The listing builds one solid part. Answer for the finished solid, in the listing's coordinates (mm). Face numbers are marked on the shaded views. A direction names the side the tool comes from. Coordinates: 2 decimals unless noted, no trailing zeros. Order: outer loops, then holes, each group sorted by start corner. A loop starts at its lowest first (then second) coordinate and runs counter-clockwise, first axis right, second up. Notation, with made-up numbers: (-28, 15.5) -> (-17, 15.5) arc R28 ccw to (-17, 53.5) -> close; hole circle Ø11 at (86, -38). An arc over 180 degrees is marked (long way). Return JSON: item names as keys, results as strings.
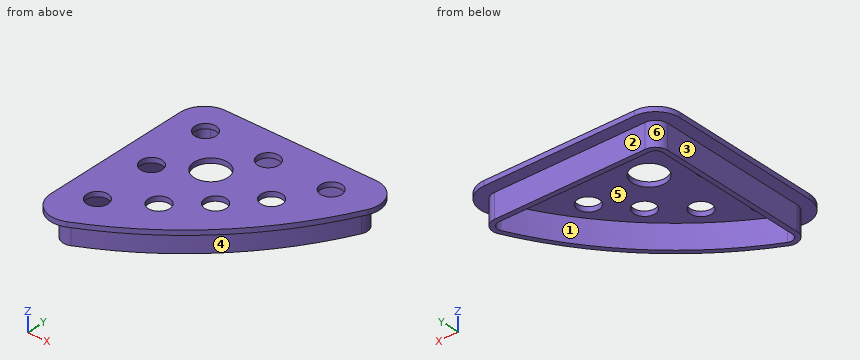
from build123d import *

# Parameters (mm, degrees)
F1_DEPTH = 12.7
F3_DEPTH = 2.54
F4_R     = 5.588
F4_R_2   = 8.763
F5_DEPTH = 25.4


with BuildPart() as f1:
    # F0 (on Top) → F1 (new body)
    with BuildSketch(Plane.XY):
        with BuildLine():
            ThreePointArc((0.508, -85.5526443698), (3.4826484531, -90.931259613), (9.6196541528, -91.2706655607))
            ThreePointArc((9.6196541528, -91.2706655607), (57.3578547677, -57.3578547677), (91.2706655607, -9.6196541528))
            ThreePointArc((91.2706655607, -9.6196541528), (90.931259613, -3.4826484531), (85.5526443698, -0.508))
            Line((85.5526443698, -0.508), (6.858, -0.508))
            ThreePointArc((6.858, -0.508), (2.3678719395, -2.3678719395), (0.508, -6.858))
            Line((0.508, -6.858), (0.508, -85.5526443698))
        make_face()
        with BuildLine():
            ThreePointArc((88.9834570843, -8.5149924917), (55.5618035435, -55.5618035435), (8.5149924917, -88.9834570843))
            ThreePointArc((8.5149924917, -88.9834570843), (4.8327890719, -88.7798135157), (3.048, -85.5526443698))
            Line((3.048, -85.5526443698), (3.048, -6.858))
            ThreePointArc((3.048, -6.858), (4.1639231637, -4.1639231637), (6.858, -3.048))
            Line((6.858, -3.048), (85.5526443698, -3.048))
            ThreePointArc((85.5526443698, -3.048), (88.7798135157, -4.8327890719), (88.9834570843, -8.5149924917))
        make_face(mode=Mode.SUBTRACT)
    extrude(amount=F1_DEPTH)

    # F2 (on face) → F3 (join)
    with BuildSketch(Plane.XY.offset(12.7)):
        with BuildLine():
            Line((85.5526443698, 5.842), (6.858, 5.842))
            ThreePointArc((6.858, 5.842), (-2.1222561211, 2.1222561211), (-5.842, -6.858))
            Line((-5.842, -6.858), (-5.842, -85.5526443698))
            ThreePointArc((-5.842, -85.5526443698), (0.1072969063, -96.3098748563), (12.3813083055, -96.9886867517))
            ThreePointArc((12.3813083055, -96.9886867517), (61.8479828282, -61.8479828282), (96.9886867517, -12.3813083055))
            ThreePointArc((96.9886867517, -12.3813083055), (96.3098748563, -0.1072969063), (85.5526443698, 5.842))
        make_face()
        with BuildLine():
            ThreePointArc((9.6196541528, -91.2706655607), (3.4826484531, -90.931259613), (0.508, -85.5526443698))
            Line((0.508, -85.5526443698), (0.508, -6.858))
            ThreePointArc((0.508, -6.858), (2.3678719395, -2.3678719395), (6.858, -0.508))
            Line((6.858, -0.508), (85.5526443698, -0.508))
            ThreePointArc((85.5526443698, -0.508), (90.931259613, -3.4826484531), (91.2706655607, -9.6196541528))
            ThreePointArc((91.2706655607, -9.6196541528), (57.3578547677, -57.3578547677), (9.6196541528, -91.2706655607))
        make_face(mode=Mode.SUBTRACT)
        with BuildLine():
            Line((0.508, -6.858), (0.508, -85.5526443698))
            ThreePointArc((0.508, -85.5526443698), (3.4826484531, -90.931259613), (9.6196541528, -91.2706655607))
            ThreePointArc((9.6196541528, -91.2706655607), (57.3578547677, -57.3578547677), (91.2706655607, -9.6196541528))
            ThreePointArc((91.2706655607, -9.6196541528), (90.931259613, -3.4826484531), (85.5526443698, -0.508))
            Line((85.5526443698, -0.508), (6.858, -0.508))
            ThreePointArc((6.858, -0.508), (2.3678719395, -2.3678719395), (0.508, -6.858))
        make_face()
        with BuildLine():
            ThreePointArc((85.5526443698, -3.048), (88.7798135157, -4.8327890719), (88.9834570843, -8.5149924917))
            ThreePointArc((88.9834570843, -8.5149924917), (55.5618035435, -55.5618035435), (8.5149924917, -88.9834570843))
            ThreePointArc((8.5149924917, -88.9834570843), (4.8327890719, -88.7798135157), (3.048, -85.5526443698))
            Line((3.048, -85.5526443698), (3.048, -6.858))
            ThreePointArc((3.048, -6.858), (4.1639231637, -4.1639231637), (6.858, -3.048))
            Line((6.858, -3.048), (85.5526443698, -3.048))
        make_face(mode=Mode.SUBTRACT)
        with BuildLine():
            ThreePointArc((8.5149924917, -88.9834570843), (55.5618035435, -55.5618035435), (88.9834570843, -8.5149924917))
            ThreePointArc((88.9834570843, -8.5149924917), (88.7798135157, -4.8327890719), (85.5526443698, -3.048))
            Line((85.5526443698, -3.048), (6.858, -3.048))
            ThreePointArc((6.858, -3.048), (4.1639231637, -4.1639231637), (3.048, -6.858))
            Line((3.048, -6.858), (3.048, -85.5526443698))
            ThreePointArc((3.048, -85.5526443698), (4.8327890719, -88.7798135157), (8.5149924917, -88.9834570843))
        make_face()
    extrude(amount=F3_DEPTH)

    # F4 (on face) → F5 (cut)
    with BuildSketch(Plane.XY.offset(15.24)):
        with Locations((10.7421888637, -10.7421888637)):
            Circle(F4_R)
        with Locations((30.9239914141, -30.9239914141)):
            Circle(F4_R_2)
        with Locations((43.5884171282, -10.7421888637)):
            Circle(F4_R)
        with Locations((10.7421888637, -43.5884171282)):
            Circle(F4_R)
        with Locations((10.7421888637, -76.4346453927)):
            Circle(F4_R)
        with Locations((31.4632623863, -63.1055415565)):
            Circle(F4_R)
        with Locations((48.3775986466, -48.3775986466)):
            Circle(F4_R)
        with Locations((63.1055415565, -31.4632623863)):
            Circle(F4_R)
        with Locations((76.4346453927, -10.7421888637)):
            Circle(F4_R)
    extrude(amount=-F5_DEPTH, mode=Mode.SUBTRACT)


solid = f1.part
1. The part is cut by section C-C on y = -45.5. Give the vertices of the cut face in (x, z).
Answer block:
{"outline": "(-5.84, 12.7) -> (0.51, 12.7) -> (0.51, 0) -> (3.05, 0) -> (3.05, 12.7) -> (5.49, 12.7) -> (5.49, 15.24) -> (-5.84, 15.24) -> close; (15.99, 12.7) -> (43.59, 12.7) -> (43.59, 15.24) -> (15.99, 15.24) -> close; (53.17, 12.7) -> (64.86, 12.7) -> (64.86, 0) -> (68.18, 0) -> (68.18, 12.7) -> (76.34, 12.7) -> (76.34, 15.24) -> (53.17, 15.24) -> close"}
2. Each of these flat-tipped pins is pushed along its axis until it touches: pin 1 Ø2 at (x, z) = (45, 8) entering from -Y; pin 2 Ø6.5 at (y, z) = (-29.5, 7) entering from -X; pin 3 Ø14.5 at (x, y) = (48.38, -48.38) entering from -Z. Where does it stop, or does it pass through?
Answer block:
{"pin 1": "stops at y = -69.41", "pin 2": "stops at x = 0.51", "pin 3": "stops at z = 12.7"}
3. The part is cut by section A-A on z = 5.5. Give the vertices of the cut face in (x, y) (3 decimals).
Answer block:
{"outline": "(0.508, -85.553) arc R6.35 ccw to (9.62, -91.271) arc R175.379 ccw to (91.271, -9.62) arc R6.35 ccw to (85.553, -0.508) -> (6.858, -0.508) arc R6.35 ccw to (0.508, -6.858) -> close; hole (3.048, -85.553) arc R3.81 ccw to (8.515, -88.983) arc R172.839 ccw to (88.983, -8.515) arc R3.81 ccw to (85.553, -3.048) -> (6.858, -3.048) arc R3.81 ccw to (3.048, -6.858) -> close"}
4. For the marked faces 1, 2 and 3, determine the directions among +Z, -Z, +X, -X, +Y, -Y from which every point of the face is accessible in a straight line to the end or side of a thin tool.
Answer block:
{"face 1": "-Z", "face 2": "-Z, +X, -X, +Y", "face 3": "-Z, -X, +Y, -Y"}
5. Consider line 1 (Z direction, x = 18, y = -38.5); line 2 (X direction, y = -42.5, z = 12.75); line 3 (X direction, y = -14, z = 1.5). Determine where each line is inside the solid, lowest interval first. Write a range as from..to.
Answer block:
{"line 1": "z = 12.7..15.24", "line 2": "x = -5.84..5.26, 16.22..78.64", "line 3": "x = 0.51..3.05, 86.21..89.08"}
6. The part is cut by section B-B on x = 50.5. Give the vertices of the cut face in (y, z).
Answer block:
{"outline": "(-72.27, 12.7) -> (-63.86, 12.7) -> (-63.86, 0) -> (-60.42, 0) -> (-60.42, 12.7) -> (-53.55, 12.7) -> (-53.55, 15.24) -> (-72.27, 15.24) -> close; (-43.21, 12.7) -> (-3.05, 12.7) -> (-3.05, 0) -> (-0.51, 0) -> (-0.51, 12.7) -> (5.84, 12.7) -> (5.84, 15.24) -> (-43.21, 15.24) -> close"}
7. Determine the mould class of the marked faces 4, 5 and 6 for opening direction X: pulls with the +X half, pulls with the -X half, needs draft (parallel to the pull), parting line crosses it, or undercut.
Answer block:
{"face 4": "pulls with the +X half", "face 5": "undercut", "face 6": "pulls with the -X half"}
8. The part is cut by section D-D on y = -35. Give the vertices of the cut face in (x, z), and give its area (3 significant figures).
Answer block:
{"outline": "(-5.84, 12.7) -> (0.51, 12.7) -> (0.51, 0) -> (3.05, 0) -> (3.05, 12.7) -> (23.17, 12.7) -> (23.17, 15.24) -> (-5.84, 15.24) -> close; (38.68, 12.7) -> (58.78, 12.7) -> (58.78, 15.24) -> (38.68, 15.24) -> close; (67.43, 12.7) -> (73.13, 12.7) -> (73.13, 0) -> (76.26, 0) -> (76.26, 12.7) -> (83.98, 12.7) -> (83.98, 15.24) -> (67.43, 15.24) -> close", "area": "239 mm2"}
